Work out the finished part from the listing and answer in its coordinate system (mm). A direction names the side the tool comes from. Round coordinates to 2 decimals unless told otherwise and drop trailing zeros. Write each loop counter-clockwise with the first axis right and the second up, starting at its lowest first coordinate (ties: lowest second). Pieces come first, ordered by that corner, then holes.
1. Find section A-A (z = 3). Write down the section's boundary in (x, y), and give its area (3 significant figures).
2. Straight lines are drawn through the part: probe 1 along X at (y, z) = (1.25, 4.5); probe 2 along Z at (x, y) = (0, -2.15); probe 3 along Y at (x, z) = (17.5, 0.45). For each, find the intervals that lie inside material, in ascending order.
3. Determine the mould class of faces 1 (the face through (19, 1, 2)), 2 (the face through (0, 5, 1)), 3 (the face through (5, 0.4, 4)) for opening direction Y: pulls with the +Y half, pulls with the -Y half, needs draft (parallel to the pull), parting line crosses it, or undercut.
4. Find section B-B (x = 0). Write down the section's boundary in (y, z), and give its area (3 significant figures).
5. Flat-ended cylindrical pins translate along their axes: pin 1 Ø4 at (x, y) = (-17.5, 0) entering from +Z; pin 2 Ø3 at (x, y) = (10, 2) entering from +Z; pin 3 Ø2 at (x, y) = (-5, -2) entering from +Z; pin 4 Ø5 at (x, y) = (-1, -0.5) entering from -Z. Find the tip coordinate at first contact, or state that the pin passes through.
6. Find section D-D (x = 17.5). Write down the section's boundary in (y, z), and give its area (3 significant figures).
7. A tool of negligible diameter and unlimited length cuts with its end or side. For faces 4 (the face through (-19, 0, 1)), 5 (the face through (-17, 3, 5)), 6 (the face through (-1.73, -2.34, 2.19)), from which of +Z, -Z, +X, -X, +Y, -Y can it reach the whole face along a straight path? Write none if from no direction.
8. Find section C-C (y = 3.5). Write down the section's boundary in (x, z).
```python
from build123d import *

# Parameters (mm, degrees)
PAD_DEPTH        = 5
HOLE_D           = 15
HOLE_CBORE_D     = 16
HOLE_CBORE_DEPTH = 5.4
SKETCH002_R      = 1.5
HOLE001_DEPTH    = 25
POCKET_DEPTH     = 18


with BuildPart() as part:
    # Sketch → Pad (new body, symmetric)
    with BuildSketch(Plane.XZ):
        with BuildLine():
            Line((-25, 0), (25, 0))
            Line((8.955135, 17.987838), (25, 0))
            ThreePointArc((8.955135, 17.987838), (0, 22), (-8.955135, 17.987838))
            Line((-8.955135, 17.987838), (-25, 0))
        make_face()
    extrude(amount=PAD_DEPTH, both=True)

    # Hole (through all)
    with Locations(Plane.XZ.offset(5)):
        with Locations((0, 10)):
            CounterBoreHole(HOLE_D / 2, HOLE_CBORE_D / 2, HOLE_CBORE_DEPTH)

    # Sketch002 (on Face6 of Hole) → Hole001 (cut)
    with BuildSketch(Plane(origin=(0, 0, 0), x_dir=(1, 0, 0), z_dir=(0, 0, -1))):
        with Locations((-17.5, 0)):
            Circle(SKETCH002_R)
        with Locations((17.5, 0)):
            Circle(SKETCH002_R)
    extrude(amount=-HOLE001_DEPTH, mode=Mode.SUBTRACT)

    # Sketch003 → Pocket (cut)
    with BuildSketch(Plane.XY.offset(20)):
        Polygon((-15.767949, 3), (-19.232051, 3), (-20.964102, 0), (-19.232051, -3), (-15.767949, -3), (-14.035898, 0), align=None)
        Polygon((15.767949, 3), (14.035898, 0), (15.767949, -3), (19.232051, -3), (20.964102, 0), (19.232051, 3), align=None)
    extrude(amount=-POCKET_DEPTH, mode=Mode.SUBTRACT)


solid = part.part
```
Worked answers:
1. outline: (-22.32, -5) - (-3.87, -5) - (-3.87, 0.4) - (-2.69, 0.4) - (-2.69, 5) - (-22.32, 5) - close; (2.69, 0.4) - (3.87, 0.4) - (3.87, -5) - (22.32, -5) - (22.32, 5) - (2.69, 5) - close; hole (-20.96, 0) - (-19.23, -3) - (-15.77, -3) - (-14.04, 0) - (-15.77, 3) - (-19.23, 3) - close; hole (14.04, 0) - (15.77, -3) - (19.23, -3) - (20.96, 0) - (19.23, 3) - (15.77, 3) - close
1. area: 318 mm2
2. probe 1: x = -20.99 to -20.24, -14.76 to -5.1, 5.1 to 14.76, 20.24 to 20.99
2. probe 2: z = 0 to 2, 18 to 22
2. probe 3: y = -5 to -1.5, 1.5 to 5
3. face 1: undercut
3. face 2: pulls with the +Y half
3. face 3: pulls with the -Y half
4. outline: (-5, 0) - (5, 0) - (5, 2.5) - (0.4, 2.5) - (0.4, 2) - (-5, 2) - close; (-5, 18) - (0.4, 18) - (0.4, 17.5) - (5, 17.5) - (5, 22) - (-5, 22) - close
4. area: 64.6 mm2
5. pin 1: stops at z = 2
5. pin 2: stops at z = 18.47
5. pin 3: stops at z = 21.31
5. pin 4: stops at z = 0
6. outline: (-5, 0) - (-1.5, 0) - (-1.5, 2) - (-3, 2) - (-3, 8.41) - (-5, 8.41) - close; (1.5, 0) - (5, 0) - (5, 8.41) - (3, 8.41) - (3, 2) - (1.5, 2) - close
6. area: 39.6 mm2
7. face 4: +Z, -Z
7. face 5: +Z
7. face 6: -Y
8. outline: (-25, 0) - (25, 0) - (8.96, 17.99) arc R12 ccw to (-8.96, 17.99) - close; hole circle Ø15 at (0, 10)
